```python
from build123d import *

# Parameters (mm, degrees)
BOSS_EXTRUDE1_DEPTH = 5
CIRPATTERN4_COUNT   = 15
SKETCH6_R           = 6.25
BOSS_EXTRUDE2_DEPTH = 5
SKETCH7_R           = 4
SKETCH7_W           = 3
SKETCH7_H           = 3
CUT_EXTRUDE1_DEPTH  = 14.011467857


with BuildPart() as part:
    # Sketch3 → Boss-Extrude1 (new body)
    with BuildSketch(Plane(origin=(0, 0, 0), x_dir=(1, 0, 0), z_dir=(0, 1, 0))):
        with BuildLine():
            Line((1.567279433, 7.07287775), (1.352139221, 6.101984884))
            ThreePointArc((1.352139221, 6.101984884), (0.680108254, 6.212886025), (0, 6.25))
            Line((0, 6.25), (0, 7.244443697))
            ThreePointArc((0, 7.244443697), (0.202974195, 7.888710473), (0.522323902, 8.483936453))
            ThreePointArc((0.522323902, 8.483936453), (0.924947225, 8.449524994), (1.325480107, 8.396017061))
            ThreePointArc((1.325480107, 8.396017061), (1.508494299, 7.745798629), (1.567279433, 7.07287775))
        make_face()
    extrude(amount=BOSS_EXTRUDE1_DEPTH)


with BuildPart() as cirpattern4_1:
    # CirPattern4: pattern copy
    add(part.part.rotate(Axis((0, 0, 0), (0, 1, 0)), 1 * 360 / CIRPATTERN4_COUNT))


with BuildPart() as cirpattern4_2:
    # CirPattern4: pattern copy
    add(part.part.rotate(Axis((0, 0, 0), (0, 1, 0)), 2 * 360 / CIRPATTERN4_COUNT))


with BuildPart() as cirpattern4_3:
    # CirPattern4: pattern copy
    add(part.part.rotate(Axis((0, 0, 0), (0, 1, 0)), 3 * 360 / CIRPATTERN4_COUNT))


with BuildPart() as cirpattern4_4:
    # CirPattern4: pattern copy
    add(part.part.rotate(Axis((0, 0, 0), (0, 1, 0)), 4 * 360 / CIRPATTERN4_COUNT))


with BuildPart() as cirpattern4_5:
    # CirPattern4: pattern copy
    add(part.part.rotate(Axis((0, 0, 0), (0, 1, 0)), 5 * 360 / CIRPATTERN4_COUNT))


with BuildPart() as cirpattern4_6:
    # CirPattern4: pattern copy
    add(part.part.rotate(Axis((0, 0, 0), (0, 1, 0)), 6 * 360 / CIRPATTERN4_COUNT))


with BuildPart() as cirpattern4_7:
    # CirPattern4: pattern copy
    add(part.part.rotate(Axis((0, 0, 0), (0, 1, 0)), 7 * 360 / CIRPATTERN4_COUNT))


with BuildPart() as cirpattern4_8:
    # CirPattern4: pattern copy
    add(part.part.rotate(Axis((0, 0, 0), (0, 1, 0)), 8 * 360 / CIRPATTERN4_COUNT))


with BuildPart() as cirpattern4_9:
    # CirPattern4: pattern copy
    add(part.part.rotate(Axis((0, 0, 0), (0, 1, 0)), 9 * 360 / CIRPATTERN4_COUNT))


with BuildPart() as cirpattern4_10:
    # CirPattern4: pattern copy
    add(part.part.rotate(Axis((0, 0, 0), (0, 1, 0)), 10 * 360 / CIRPATTERN4_COUNT))


with BuildPart() as cirpattern4_11:
    # CirPattern4: pattern copy
    add(part.part.rotate(Axis((0, 0, 0), (0, 1, 0)), 11 * 360 / CIRPATTERN4_COUNT))


with BuildPart() as cirpattern4_12:
    # CirPattern4: pattern copy
    add(part.part.rotate(Axis((0, 0, 0), (0, 1, 0)), 12 * 360 / CIRPATTERN4_COUNT))


with BuildPart() as cirpattern4_13:
    # CirPattern4: pattern copy
    add(part.part.rotate(Axis((0, 0, 0), (0, 1, 0)), 13 * 360 / CIRPATTERN4_COUNT))


with BuildPart() as cirpattern4_14:
    # CirPattern4: pattern copy
    add(part.part.rotate(Axis((0, 0, 0), (0, 1, 0)), 14 * 360 / CIRPATTERN4_COUNT))


with BuildPart() as part_1:
    add(part.part)

    add(cirpattern4_1.part)  # Boss-Extrude2 merges CirPattern4_1

    add(cirpattern4_2.part)  # Boss-Extrude2 merges CirPattern4_2

    add(cirpattern4_3.part)  # Boss-Extrude2 merges CirPattern4_3

    add(cirpattern4_4.part)  # Boss-Extrude2 merges CirPattern4_4

    add(cirpattern4_5.part)  # Boss-Extrude2 merges CirPattern4_5

    add(cirpattern4_6.part)  # Boss-Extrude2 merges CirPattern4_6

    add(cirpattern4_7.part)  # Boss-Extrude2 merges CirPattern4_7

    add(cirpattern4_8.part)  # Boss-Extrude2 merges CirPattern4_8

    add(cirpattern4_9.part)  # Boss-Extrude2 merges CirPattern4_9

    add(cirpattern4_10.part)  # Boss-Extrude2 merges CirPattern4_10

    add(cirpattern4_11.part)  # Boss-Extrude2 merges CirPattern4_11

    add(cirpattern4_12.part)  # Boss-Extrude2 merges CirPattern4_12

    add(cirpattern4_13.part)  # Boss-Extrude2 merges CirPattern4_13

    add(cirpattern4_14.part)  # Boss-Extrude2 merges CirPattern4_14
    # Sketch6 → Boss-Extrude2 (add)
    with BuildSketch(Plane(origin=(0, 0, 0), x_dir=(1, 0, 0), z_dir=(0, 1, 0))):
        Circle(SKETCH6_R)
    extrude(amount=BOSS_EXTRUDE2_DEPTH)

    # Sketch7 → Cut-Extrude1 (cut, through all)
    with BuildSketch(Plane(origin=(0, 5, 0), x_dir=(1, 0, 0), z_dir=(0, 1, 0))):
        Circle(SKETCH7_R)
        with Locations((0, 4)):
            Rectangle(SKETCH7_W, SKETCH7_H)
    extrude(amount=-CUT_EXTRUDE1_DEPTH, mode=Mode.SUBTRACT)


solid = part_1.part
```
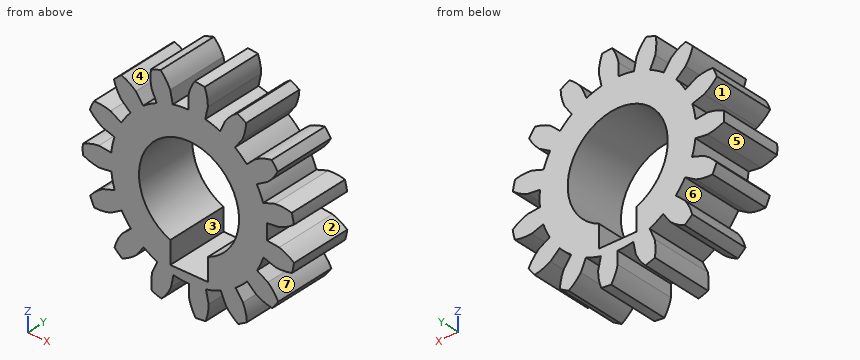
Check sheet for the modelled part. Datum: model origin and axes. Units: mm. Face numbers are marked on the shaded views. A direction names the side the tool comes from. Round coordinates to 2 decimals unless told otherwise and drop trailing zeros. Loops run counter-clockwise (first coordinate to the right, second up) from the corner with the lowest first, then second, coordinate; pieces in that order, holes last. Notation, with made-up numbers: (50, 64.5) - (71, 64.5) arc R22 cw to (71, 85.5) - close; hole circle Ø9 at (53, 55). An arc over 180 degrees is marked (long way). Answer as a JSON object with one key per item and string values. Group by question number.
Q1. Gauge pin test, flat ends, axial feed: P1, Ø0.5, axis at y = 2, z = -6.5, coming from the -X side; P2, Ø2, axis at x = -0.5, y = 4, coming from the +Z side; P3, Ø0.5, axis at y = 2, z = -4.5, coming from the +X side; P4, Ø3, axis at x = 4, y = 2.5, coming from the -Z side. Record the tip position at first contact, or that the pin passes through.
Q2. Scan lines: line 1 along X through (y, z) = (3.3, -7.25); line 2 along X through (y, z) = (1.85, 0); line 3 along Z through (x, y) = (-0.75, 3.8). Record each from-to range of solid material in increasing order. Write a range as [from, to].
Q3. Mould release check, pull along X, two halves, no side actions. Record for the marked faces 1, 2 and 3: released by +X, released by -X, zero draft, split by the parting line, or undercut.
Q4. Set-up check for the marked faces 4, 5, 6 and 7: record each of +Z, -Z, +X, -X, +Y, -Y from which the full face is reachable in a straight line by a thin tool's end or side.
Q5. Sectioned sample at A-A, the plane z = 0. Enter the section's corners in (x, y), plus the area to 4 significant figures.
Solution:
{
 "1": {"P1": "stops at x = -5.76", "P2": "stops at z = 8.49", "P3": "stops at x = 7.13", "P4": "stops at z = -7.54"},
 "2": {"line 1": "x = [-3.02, -1.52], [0, 1.56], [3.54, 4.44]", "line 2": "x = [-8.5, -4], [4, 6.25]", "line 3": "z = [-6.2, -5.5], [3.93, 6.2]"},
 "3": {"face 1": "released by -X", "face 2": "released by +X", "face 3": "undercut"},
 "4": {"face 4": "+Z, +Y, -Y", "face 5": "-X, +Y, -Y", "face 6": "+Y, -Y", "face 7": "+X, +Y, -Y"},
 "5": {"outline": "(-8.5, 0) - (-4, 0) - (-4, 5) - (-8.5, 5) - close; (4, 0) - (6.25, 0) - (6.25, 5) - (4, 5) - close", "area": "33.75 mm²"}
}
